```python
from build123d import *

# Parameters (mm, degrees)
F1_DEPTH = 19.05
F3_DEPTH = 9.525
F4_R     = 25.4
F5_R     = 25.4
F6_R     = 25.4
F7_R     = 25.4


# Not quite as in the source:
# - a length typed as a fraction of an inch, garbled in the dataset ("3 / 203.2 mm" for 3/8 in), is restored


with BuildPart() as f1:
    # F0 (on Front) → F1 (new body)
    with BuildSketch(Plane.XZ):
        Polygon((457.2, 163.4292998382), (0, 163.4292998382), (-457.2, 163.4292998382), (-457.2, -141.3707001618), (0, -141.3707001618), (457.2, -141.3707001618), align=None)
    extrude(amount=F1_DEPTH)

    # F2 (on Front) → F3 (cut)
    with BuildSketch(Plane.XZ):
        Polygon((425.45, -106.4507083202), (425.45, 13.6912916798), (425.45, 133.8332916798), (406.4, 133.8332916798), (406.4, 23.3432916798), (406.4, 13.6912916798), (406.4, 4.0392916798), (406.4, -106.4507083202), align=None)
        Polygon((406.4, 13.6912916798), (406.4, 23.3432916798), (-406.4, 23.3432916798), (-406.4, 13.6912916798), (-406.4, 4.0392916798), (406.4, 4.0392916798), align=None)
        Polygon((-406.4, 13.6912916798), (-406.4, 23.3432916798), (-406.4, 133.8332916798), (-425.45, 133.8332916798), (-425.45, 13.6912916798), (-425.45, -106.4507083202), (-406.4, -106.4507083202), (-406.4, 4.0392916798), align=None)
    extrude(amount=F3_DEPTH, mode=Mode.SUBTRACT)

    # F4
    f4_edges = [f1.edges().sort_by_distance(p)[0] for p in [
        (457.2, -9.525, 163.4293),
    ]]
    fillet(f4_edges, radius=F4_R)

    # F5
    f5_edges = [f1.edges().sort_by_distance(p)[0] for p in [
        (457.2, -9.525, -141.3707),
    ]]
    fillet(f5_edges, radius=F5_R)

    # F6
    f6_edges = [f1.edges().sort_by_distance(p)[0] for p in [
        (-457.2, -9.525, 163.4293),
    ]]
    fillet(f6_edges, radius=F6_R)

    # F7
    f7_edges = [f1.edges().sort_by_distance(p)[0] for p in [
        (-457.2, -9.525, -141.3707),
    ]]
    fillet(f7_edges, radius=F7_R)


solid = f1.part
```
Could you check a few things on this model? Use its own coordinates, in mm. Round coordinates to 2 decimals unless told otherwise and drop trailing zeros. Loops run counter-clockwise (first coordinate to the right, second up) from the corner with the lowest first, then second, coordinate; pieces in that order, holes last. Notation, with made-up numbers: M -14.5,5.5 L 30.5,5.5 A23 cw 30.5,13.5 Z; hole C 41,60.25 d2. An arc over 180 degrees is marked long. Put each result on its own line as item: value.
Q1. I need wall thicknesses on probe 1 along X at (y, z) = (-8, -106); probe 2 along Z at (x, y) = (117, -6.25); probe 3 along Z at (x, y) = (-416.5, -6.75). Which ranges of each line are inside material? Lowest first, please.
Check result:
probe 1: -457.2 to -425.45, -406.4 to 406.4, 425.45 to 457.2
probe 2: -141.37 to 4.04, 23.34 to 163.43
probe 3: -141.37 to -106.45, 133.83 to 163.43
Q2. Imagine slicing it at C-C (z = 32.5). Write out the boundary of the cut face in (x, y) (3 decimals).
Check result:
outline: M -457.2,-19.05 L 457.2,-19.05 L 457.2,0 L 425.45,0 L 425.45,-9.525 L 406.4,-9.525 L 406.4,0 L -406.4,0 L -406.4,-9.525 L -425.45,-9.525 L -425.45,0 L -457.2,0 Z
Q3. Thinking about a two-plate mould opening in X: for faces 1 (the face through (457.2, -9, 9)), 2 (the face through (-6, -19.05, 13)), 3 (the face through (-2, -9.525, 14)), which applies, released by +X, released by -X, zero draft, split by the parting line, or undercut?
Check result:
face 1: released by +X
face 2: zero draft
face 3: undercut
Q4. Imagine slicing it at B-B (x = -391.5). Write out the boundary of the cut face in (y, z) (3 decimals).
Check result:
outline: M -19.05,-141.371 L 0,-141.371 L 0,4.039 L -9.525,4.039 L -9.525,23.343 L 0,23.343 L 0,163.429 L -19.05,163.429 Z
Q5. Imagine slicing it at A-A (y = -5.5). Write out the boundary of the cut face in (x, z).
Check result:
outline: M -457.2,-115.97 A25.4 ccw -431.8,-141.37 L 431.8,-141.37 A25.4 ccw 457.2,-115.97 L 457.2,138.03 A25.4 ccw 431.8,163.43 L -431.8,163.43 A25.4 ccw -457.2,138.03 Z; hole M -425.45,-106.45 L -406.4,-106.45 L -406.4,4.04 L 406.4,4.04 L 406.4,-106.45 L 425.45,-106.45 L 425.45,133.83 L 406.4,133.83 L 406.4,23.34 L -406.4,23.34 L -406.4,133.83 L -425.45,133.83 Z
